Study the drawing (mm; zero at the part's minimum x, y, z) and answer. Give positions to 0.01 mm unless a question says otherwise; leave off trailing zeros. Order: outer loops, then holes, each group sorted by start corner. A loop starts at its lowest first (then second) coordinate and runs counter-clockwise, first axis right, second up. Notation, with made-up numbers: (48.25, -12.75) -> (95.25, -12.75) arc R26 ccw to (95.25, 22.25) -> close; hole circle Ø6 at (-1.5, -11.75). An arc over 180 degrees is marked (long way). Answer as CSV lines item,"result". Start each with the question number.
1. Flat-ended cylindrical pins translate along their axes: pin 1 (3 mm diameter, centred on x = 9, z = 5.5, fed in from -Y); pin 2 (8 mm diameter, centred on x = 15, y = 12.5, fed in from -Z); pin 3 (3 mm diameter, centred on y = 3, z = 7, fed in from -X) (1 decimal). Find the tip coordinate at first contact, or state that the pin passes through.
2. Find the intervals of material crossed by L1, parallel to X at y = 13, z = 6.5; L2, parallel to X at y = 10.75, z = 5; L3, parallel to Y at x = 8.25, z = 6.75 (1 decimal), in increasing order.
3. For a pull along Y with two mould halves and no side action, classify the marked faces 1, 2, 3 and 4 as released by +Y, released by -Y, zero draft, split by the parting line, or undercut.
4. A cutting plane is placed at A-A (z = 6.75). Give the vertices of the cut face in (x, y) (1 decimal), then the cut area to 3 significant figures.
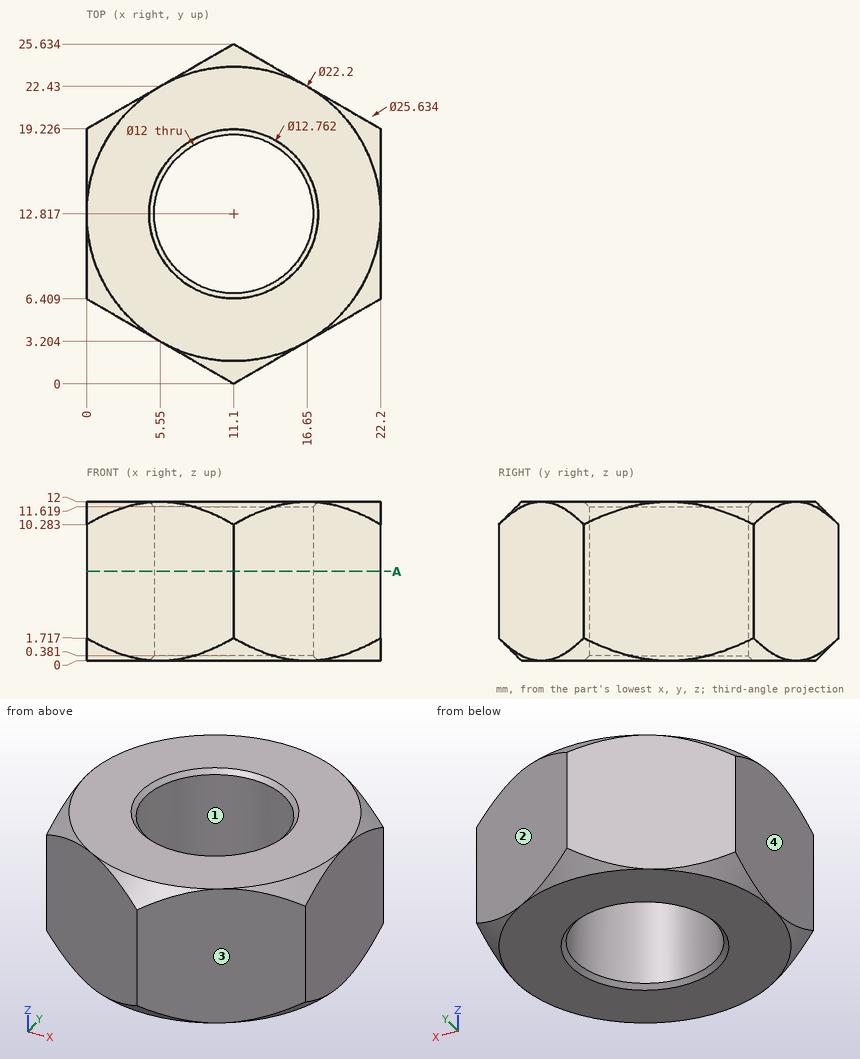
Answer sheet:
1,pin 1,"stops at y = 0.35"
1,pin 2,"stops at z = 0"
1,pin 3,"stops at x = 3.3"
2,L1,"x = 0 to 5.1, 17.1 to 22.2"
2,L2,"x = 0 to 5.47, 16.73 to 22.2"
2,L3,"y = 1.6 to 7.5, 18.1 to 24"
3,face 1,"undercut"
3,face 2,"released by +Y"
3,face 3,"released by -Y"
3,face 4,"zero draft"
4,outline,"(0, 6.4) -> (11.1, 0) -> (22.2, 6.4) -> (22.2, 19.2) -> (11.1, 25.6) -> (0, 19.2) -> close; hole circle Ø12 at (11.1, 12.8)"
4,area,"314 mm^2"
